Autodesk Inventor part; units mm, degrees
ref_plane "YZ Plane" through (0, 0, 0) normal (1, 0, 0) x (0, 1, 0)
ref_plane "XZ Plane" through (0, 0, 0) normal (0, 1, 0) x (-1, 0, 0)
ref_plane "XY Plane" through (0, 0, 0) normal (0, 0, 1) x (1, 0, 0)
sketch "Sketch1" plane through (0, 0, 0) normal (0, 1, 0) x (-1, 0, 0)
  line L0 (19.5, 15.5) -> (-19.5, 15.5)
  line L1 (-19.5, -15.5) -> (19.5, -15.5)
  line L2 (19.5, -15.5) -> (19.5, 15.5)
  line L3 (24, -20) -> (-24, -20)
  line L4 (-24, 20) -> (24, 20)
  line L5 (24, 20) -> (24, -20)
  line L6 (-19.5, -3.5) -> (-24, -3.5)
  line L7 (-19.5, 3.5) -> (-24, 3.5)
  line L8 (-19.5, -3.5) -> (-19.5, -15.5)
  line L9 (-24, -20) -> (-24, -3.5)
  line L10 (-24, 3.5) -> (-24, 20)
  line L11 (-19.5, 3.5) -> (-19.5, 15.5)
  circle A0 centre (24, -20) radius 4
  circle A1 centre (24, 20) radius 4
  circle A2 centre (-24, 20) radius 4
  circle A3 centre (-24, -20) radius 4
  point P0 (0, 0)
  point P1 (0, -15.5)
  point P2 (19.5, 0)
  point P3 (0, 20)
  point P4 (24, 0)
  dimension "d0" = 39
  dimension "d1" = 31
  dimension "d2" = 4.5
  dimension "d25" = 4.5
  dimension "d27" = 4.5
  dimension "d28" = 16.5
  dimension "d29" = 8
  dimension "d30" = 8
  dimension "d31" = 8
  dimension "d32" = 8
extrude "Extrusion1" add sketch "Sketch1" along normal blind 5
sketch "Sketch2" plane through (0, 0, 0) normal (0, -1, 0) x (1, 0, 0)
  line L0 (-19.5, -15.5) -> (-19.5, 15.5)
  line L1 (-19.5, 15.5) -> (19.5, 15.5)
  line L2 (19.5, -15.5) -> (-19.5, -15.5)
  line L3 (24, -16) -> (24, -3.5)
  line L4 (20, 20) -> (-20, 20)
  line L5 (-24, 16) -> (-24, -16)
  line L6 (-20, -20) -> (20, -20)
  line L7 (19.5, -15.5) -> (-19.5, -15.5) construction
  line L8 (-40, 34) -> (40, 34) construction
  line L9 (40, 34) -> (40, -34) construction
  line L10 (40, -34) -> (-40, -34) construction
  line L11 (-40, -34) -> (-40, 34) construction
  line L12 (-40, 34) -> (-19.5, 15.5) construction
  line L13 (-40, -34) -> (-19.5, -15.5) construction
  line L14 (40, -34) -> (20, -15) construction
  line L15 (22, 18) -> (40, 34) construction
  line L16 (24, -3.5) -> (19.5, -3.5)
  line L17 (19.5, -3.5) -> (19.5, -15.5)
  line L18 (19.5, 3.5) -> (24, 3.5)
  line L19 (24, 3.5) -> (24, 16)
  line L20 (19.5, 15.5) -> (19.5, 3.5)
  arc A0 (-20, 20) -> (-24, 16) centre (-24, 20) ccw
  arc A1 (-24, -16) -> (-20, -20) centre (-24, -20) ccw
  arc A2 (20, -20) -> (24, -16) centre (24, -20) ccw
  arc A3 (24, 16) -> (20, 20) centre (24, 20) ccw
  point P0 (0, 0)
  point P1 (-40, 0)
  point P2 (0, 34)
  point P3 (-29.75, -24.75)
  point P4 (30, -24.5)
  point P5 (31, 26)
  point P6 (-29.75, 24.75)
  dimension "d14" = 54
  dimension "d15" = 64
hole "Hole1" [suppressed]
sketch "Sketch3" plane through (0, 0, 0) normal (0, -1, 0) x (1, 0, 0)
  point P0 (0, 0)
properties part number "cubierta2"
Here's how the part is built. I have some questions about the finished solid (model axes, mm). A direction names the side the tool comes from. Round coordinates to 2 decimals unless told otherwise and drop trailing zeros. Order: outer loops, then holes, each group sorted by start corner. A loop starts at its lowest first (then second) coordinate and runs counter-clockwise, first axis right, second up. Notation, with made-up numbers: M 21,4 L 45,4 A16 cw 45,30 Z; hole C -9.75,28 d8. An arc over 180 degrees is marked long. One line per question, with ' | ' between items.
1) I want a section at C-C, the plane z = -0.5. Write out the boundary of the cut face in (x, y).
Working result:
outline: M -24,0 L -19.5,0 L -19.5,5 L -24,5 Z
2) For faces 1 (the face through (22, 2, -3.5)), 2 (the face through (0, 0, -16)), 3 (the face through (-24, 2, 0)), 4 (the face through (0, 2, -20)), 5 (the face through (0, 2, -15.5)), which set-ups out of +Z, -Z, +X, -X, +Y, -Y let a thin tool reach every point of the face, with its end or its side?
Working result:
face 1: +X, +Y, -Y | face 2: +Z, -Z, +X, -X, -Y | face 3: -X, +Y, -Y | face 4: -Z, +Y, -Y | face 5: +Y, -Y
3) If we mould it in two halves opening along Z, with no side actions, what happens to faces 6 (the face through (-19.5, 2, 0)), 7 (the face through (0, 2, 20)), 8 (the face through (0, 5, -16))? For each: +Z half, -Z half, draft (parallel to the pull), parting line (faces both ways), or undercut.
Working result:
face 6: undercut | face 7: +Z half | face 8: draft
4) I want a section at A-A, the plane z = 7. Write out the boundary of the cut face in (x, y), then the cut area to 3 significant figures.
Working result:
outline: M -24,0 L -19.5,0 L -19.5,5 L -24,5 Z; M 19.5,0 L 24,0 L 24,5 L 19.5,5 Z | area: 45.0 mm²
5) I need wall thicknesses on line 1 along X through (y, z) = (2.15, -15); line 2 along Z through (x, y) = (-1.5, 2.95); line 3 along X through (y, z) = (2.9, -1). Which ranges of each line are inside material? Lowest first, please.
Working result:
line 1: -24 to -19.5, 19.5 to 24 | line 2: -20 to -15.5, 15.5 to 20 | line 3: -24 to -19.5
6) For pin 1 Ø1 at (x, y) = (11.5, 3.5) entering from -Z; pin 2 Ø1.5 at (y, z) = (1.5, 7) entering from -X; pin 3 Ø1.3 at (x, y) = (22.5, 2) entering from -Z, each with a flat end and sliding along its axis, tell me the tip position at first contact or that it passes through.
Working result:
pin 1: z = -20 | pin 2: x = -24 | pin 3: z = -23.91
7) I want a section at B-B, the plane y = 2.75. Write out the boundary of the cut face in (x, z), then the cut area to 3 significant figures.
Working result:
outline: M -24,-16 A4 ccw long -20,-20 L 20,-20 A4 ccw long 24,-16 L 24,-3.5 L 19.5,-3.5 L 19.5,-15.5 L -19.5,-15.5 L -19.5,15.5 L 19.5,15.5 L 19.5,3.5 L 24,3.5 L 24,16 A4 ccw long 20,20 L -20,20 A4 ccw long -24,16 Z | area: 830 mm²
